Autodesk Inventor part; units mm, degrees
ref_plane "YZ Plane" through (0, 0, 0) normal (1, 0, 0) x (0, 1, 0)
ref_plane "XZ Plane" through (0, 0, 0) normal (0, 1, 0) x (-1, 0, 0)
ref_plane "XY Plane" through (0, 0, 0) normal (0, 0, 1) x (1, 0, 0)
sketch "Boceto1" plane through (0, 0, 0) normal (0, 0, 1) x (1, 0, 0)
  line L0 (20, -40) -> (-20, -40)
  line L1 (-20, -40) -> (-20, 40)
  line L2 (-20, 40) -> (20, 40)
  line L3 (20, 40) -> (20, -40)
  line L4 (20, -40) -> (-20, 40) construction
  line L5 (-20, -40) -> (20, 40) construction
  point P0 (0, 0)
  dimension "d0" = 40
  dimension "d22" = 80
extrude "Extrusión1" add sketch "Boceto1" along normal blind 5
sketch "Boceto2" plane through (0, 0, 5) normal (0, 0, 1) x (1, 0, 0)
  line L0 (17.5, -37.5) -> (-17.5, -37.5)
  line L1 (-17.5, -37.5) -> (-17.5, 37.5)
  line L2 (-17.5, 37.5) -> (17.5, 37.5)
  line L3 (17.5, 37.5) -> (17.5, -37.5)
  line L4 (17.5, -37.5) -> (-17.5, 37.5) construction
  line L5 (-17.5, -37.5) -> (17.5, 37.5) construction
  line L6 (17, 37) -> (-17, 37)
  line L7 (-17, 37) -> (-17, -37)
  line L8 (-17, -37) -> (17, -37)
  line L9 (17, -37) -> (17, 37)
  line L10 (-13, 33) -> (13, 33)
  line L11 (13, 33) -> (13, -33)
  line L12 (13, -33) -> (-13, -33)
  line L13 (-13, -33) -> (-13, 33)
  line L14 (8, 33) -> (8, 37)
  line L15 (-8, 33) -> (-8, 37)
  line L16 (13, 28) -> (17, 28)
  line L17 (13, -28) -> (17, -28)
  line L18 (-13, -28) -> (-17, -28)
  line L19 (-8, -33) -> (-8, -37)
  line L20 (8, -33) -> (8, -37)
  line L21 (-17, 28) -> (-13, 28)
  point P0 (0, 0)
  dimension "d5" = 35
  dimension "d6" = 75
  dimension "d7" = 0.5
  dimension "d8" = 4
  dimension "d9" = 5
  dimension "d10" = 5
  dimension "d11" = 5
  dimension "d12" = 5
  dimension "d13" = 5
  dimension "d14" = 5
  dimension "d15" = 5
  dimension "d16" = 5
extrude "Extrusión2" add sketch "Boceto2" along normal blind 7 contours L14 L10 L15 L6 | L9 L17 L11 L16 | L21 L13 L18 L7 | L8 L19 L12 L20
fillet "Empalme3" radius 6.5 4 edges at (20, 40, 2.5) (-20, 40, 2.5) (20, -40, 2.5) (-20, -40, 2.5)
properties part number "Tapacanto Superior"
Read the model definition and answer for the solid it produces. Units are mm, in the model's axes. A direction names the side the tool comes from. Round coordinates to 2 decimals unless told otherwise and drop trailing zeros. Write each loop counter-clockwise with the first axis right and the second up, starting at its lowest first coordinate (ties: lowest second). Pieces come first, ordered by that corner, then holes. Notation, with made-up numbers: (56, 1) - (100, 1) arc R7 cw to (100, 13) - close; hole circle Ø2 at (-8.75, 49). An arc over 180 degrees is marked (long way). One line per item, written item: value.
Q1. Straight lines are drawn through the part: line 1 (Y direction, x = 4, z = 7.75); line 2 (X direction, y = -17, z = 6); line 3 (Z direction, x = -8, y = -7.5). For each, find the intervals that lie inside material, in ascending order. Write a range as from..to.
The answers:
line 1: y = -37..-33, 33..37
line 2: x = -17..-13, 13..17
line 3: z = 0..5
Q2. Each of these flat-tipped pins is pushed along its axis until it touches: P1, Ø5.5, axis at x = -0.5, z = 10, coming from the +Y side; P2, Ø2, axis at y = -35, z = 9, coming from the -X side; P3, Ø2, axis at y = -10, z = 8.5, coming from the -X side. Where does it stop, or does it pass through?
The answers:
P1: stops at y = 37
P2: stops at x = -8
P3: stops at x = -17
Q3. Which of the six approach directions +Z, -Z, +X, -X, +Y, -Y give full straight-line access (tool end or side, diameter ignored) to faces 1 (the flat face through (15, 28, 8)), 2 (the flat face through (8, 35, 8)), 3 (the flat face through (13, 0, 8)), 4 (the flat face through (15, -28, 8)), 5 (the flat face through (-8, -35, 8))?
The answers:
face 1: +Z, +X, -X, +Y
face 2: +Z, +X, +Y, -Y
face 3: +Z, +Y, -Y
face 4: +Z, +X, -X, -Y
face 5: +Z, -X, +Y, -Y
Q4. Find section C-C (y = -11). Determine the outline of the cut face in (x, z), and give its area (3 significant figures).
The answers:
outline: (-20, 0) - (20, 0) - (20, 5) - (17, 5) - (17, 12) - (13, 12) - (13, 5) - (-13, 5) - (-13, 12) - (-17, 12) - (-17, 5) - (-20, 5) - close
area: 256 mm2
Q5. For a pull along Y with two mould halves and no side action, classify faces 6 (the flat face through (0, -33, 8)), 7 (the flat face through (0, 37, 8)), 8 (the flat face through (0, -35, 12)), 9 (the flat face through (0, 33, 8)) as pulls with the +Y half, pulls with the -Y half, needs draft (parallel to the pull), parting line crosses it, or undercut.
The answers:
face 6: undercut
face 7: pulls with the +Y half
face 8: needs draft
face 9: undercut
Q6. Find section B-B (x = -4.5). Determine the outline of the cut face in (y, z), and give its area (3 significant figures).
The answers:
outline: (-40, 0) - (40, 0) - (40, 5) - (37, 5) - (37, 12) - (33, 12) - (33, 5) - (-33, 5) - (-33, 12) - (-37, 12) - (-37, 5) - (-40, 5) - close
area: 456 mm2
Q7. Find section A-A (z = 6.75). Determine the outline of the cut face in (x, y), and give its area (3 significant figures).
The answers:
outline: (-17, -28) - (-13, -28) - (-13, 28) - (-17, 28) - close; (-8, -37) - (8, -37) - (8, -33) - (-8, -33) - close; (-8, 33) - (8, 33) - (8, 37) - (-8, 37) - close; (13, -28) - (17, -28) - (17, 28) - (13, 28) - close
area: 576 mm2
Q8. Find section D-D (x = -9). Determine the outline of the cut face in (y, z), and give its area (3 significant figures).
The answers:
outline: (-40, 0) - (40, 0) - (40, 5) - (-40, 5) - close
area: 400 mm2
